from build123d import *

# Parameters (mm, degrees)
SALIENTE_EXTRUIR1_DEPTH = 150
CORTAR_EXTRUIR1_DEPTH   = 158.787979874
CORTAR_EXTRUIR2_DEPTH   = 75


with BuildPart() as part:
    # Croquis1 → Saliente-Extruir1 (new body)
    with BuildSketch(Plane.XY):
        with BuildLine():
            Line((-34.235166026, 7.276909179), (-31.300723223, 6.653174106))
            ThreePointArc((-31.300723223, 6.653174106), (0, 32), (31.300723223, 6.653174106))
            Line((31.300723223, 6.653174106), (34.235166026, 7.276909179))
            ThreePointArc((34.235166026, 7.276909179), (0, 35), (-34.235166026, 7.276909179))
        make_face()
    extrude(amount=SALIENTE_EXTRUIR1_DEPTH)

    # Croquis2 → Cortar-Extruir1 (cut, through all)
    with BuildSketch(Plane(origin=(0, 0, 0), x_dir=(1, 0, 0), z_dir=(0, 1, 0))):
        Polygon((-22.708838208, -11.554693253), (25.4976429, -11.554693253), (10.756818098, -61.753177712), (-3.585606033, -61.753177712), align=None)
    extrude(amount=CORTAR_EXTRUIR1_DEPTH, mode=Mode.SUBTRACT)

    # Croquis3 → Cortar-Extruir2 (cut, symmetric)
    with BuildSketch(Plane(origin=(0, 0, 0), x_dir=(0, 0, -1), z_dir=(1, 0, 0))):
        with BuildLine():
            Line((-11.953093924, 11.065770631), (-11.953093924, 0))
            Line((-11.953093924, 0), (-140.636510433, 0))
            Line((-140.636510433, 0), (-140.636510433, 11.065770631))
            ThreePointArc((-140.636510433, 11.065770631), (-76.294802179, 23.859279702), (-11.953093924, 11.065770631))
        make_face()
    extrude(amount=CORTAR_EXTRUIR2_DEPTH, both=True, mode=Mode.SUBTRACT)


solid = part.part
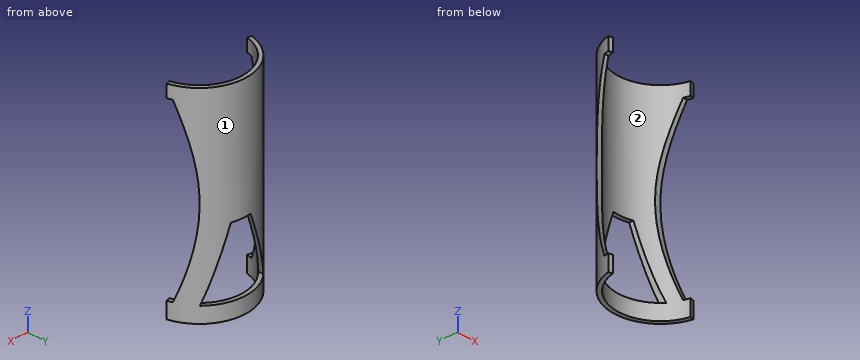
Work out the finished part from the listing and answer in its coordinate system (mm). Face numbers are marked on the shaded views. Round coordinates to 2 decimals unless told otherwise and drop trailing zeros. Loops run counter-clockwise (first coordinate to the right, second up) from the corner with the lowest first, then second, coordinate; pieces in that order, holes last. Notation, with made-up numbers: (-1, 23) -> (56, 23) arc R21 ccw to (56, 54) -> close; hole circle Ø2 at (-17.75, 54.25). An arc over 180 degrees is marked (long way). Use one line per item in the form item = value.
(1) Find section D-D on x = 23. Give the vertices of the cut face in (y, z).
Answer list:
outline = (22.25, 0) -> (26.38, 0) -> (26.38, 11.55) -> (22.25, 11.55) -> close; (22.25, 20.06) -> (26.38, 20.06) -> (26.38, 150) -> (22.25, 150) -> (22.25, 99.52) arc R168.19 cw to (22.25, 53.07) -> close
(2) Find section B-B on y = 17. Give the vertices of the cut face in (x, z).
Answer list:
outline = (-30.59, 0) -> (-27.11, 0) -> (-27.11, 28.75) -> (-30.59, 28.75) -> close; (-30.59, 123.84) -> (-27.11, 123.84) -> (-27.11, 150) -> (-30.59, 150) -> close; (27.11, 0) -> (30.59, 0) -> (30.59, 28.75) -> (27.11, 28.75) -> close; (27.11, 123.84) -> (30.59, 123.84) -> (30.59, 150) -> (27.11, 150) -> close
(3) Find section C-C on z = 23. Give the vertices of the cut face in (x, y), then the cut area to 3 significant figures.
Answer list:
outline = (-31.53, 15.19) -> (-28.16, 15.19) arc R32 cw to (-18.35, 26.22) -> (-18.35, 29.8) arc R35 ccw to start; (22.14, 23.11) arc R32 cw to (28.16, 15.19) -> (31.53, 15.19) arc R35 ccw to (22.14, 27.11) -> close
area = 90.3 mm2
(4) Flat-ended cylindrical pins translate along their axes: P1, Ø5, axis at x = 22.5, z = 73.5, coming from the +Y side; P2, Ø1.5, axis at y = 31.5, z = 127.5, coming from the +X side; P3, Ø4.5, axis at x = 5.5, y = 28, coming from the +Z side; P4, Ø5, axis at y = 29.5, z = 90, coming from the +X side. Find the tip coordinate at first contact, or state that the pin passes through.
Answer list:
P1 = 28.72
P2 = 16.72
P3 = through
P4 = 22.27
(5) Straight lines are drawn through the part: line 1 (X direction, y = 22, z = 9); line 2 (Z direction, x = -2, y = 32.25); line 3 (Y direction, x = 0.5, z = 108). For each, find the intervals that lie inside material, in ascending order.
Answer list:
line_1 = -27.22 to -23.24, 23.24 to 27.22
line_2 = 0 to 11.55, 61.75 to 150
line_3 = 32 to 35
(6) Find section A-A on x = -27. Give the vertices of the cut face in (y, z).
Answer list:
outline = (17.18, 0) -> (22.27, 0) -> (22.27, 53.24) arc R168.19 cw to (17.18, 29.35) -> close; (17.18, 123.24) arc R168.19 cw to (22.27, 99.35) -> (22.27, 150) -> (17.18, 150) -> close
(7) For a pull along X with two mould halves and no side action, classify the marked faces 1 and 2 as released by +X, released by -X, zero draft, split by the parting line, or undercut.
Answer list:
face_1 = split by the parting line
face_2 = undercut
